Source: CAD feature listing. Evaluate the final solid. Frame: model axes, mm. Face numbers are marked on the shaded views. Coordinates: 2 decimals unless noted, no trailing zeros. Write each loop counter-clockwise with the first axis right and the second up, starting at its lowest first coordinate (ties: lowest second). Pieces come first, ordered by that corner, then holes. Notation, with made-up numbers: (-4.5, -5) -> (13.5, -5) arc R18 ccw to (13.5, 6) -> close; hole circle Ø5 at (63.5, 20). An arc over 180 degrees is marked (long way). One line per item, written item: value. Start each with the question number.
1. Line query: line 1 (Y direction, x = 10, z = -1.8); line 2 (Y direction, x = 8.5, z = -4.65); line 3 (X direction, y = 63.5, z = -1.05). Output: solid intervals per line, ascending.
2. First-contact query: P1, Ø3.5, axis at x = 10, y = 87.5, coming from the +Z side. Flat tip, straight axial feed; report the tip coordinate or a pass-through.
3. Section query D-D, the plane y = 62.5. Output: boundary loops of the cut face in (x, z).
4. Section query B-B, the plane x = 10. Output: boundary loops of the cut face in (y, z), and give its area (3 significant figures).
5. Mould query, pull axis Y, two halves, no side actions, for the marked faces 1, 2, 3 and 4. Classes: released by +Y, released by -Y, zero draft, split by the parting line, or undercut.
6. Section query C-C, the plane z = -1.5. Output: boundary loops of the cut face in (x, y), and give its area (3 significant figures).
7. Section query A-A, the plane y = 12.5. Output: boundary loops of the cut face in (x, z).
from build123d import *

# Parameters (mm, degrees)
ESQUISSE1_W        = 20
ESQUISSE1_H        = 100
ESQUISSE1_R        = 4.5
ESQUISSE1_R_2      = 2.75
BOSS_EXTRU_2_DEPTH = 5


with BuildPart() as part:
    # Esquisse1 → Boss.-Extru.2 (new body)
    # profile 1 of 3: a face of its own
    with BuildSketch(Plane.XY):
        with Locations((10, 50)):
            Rectangle(ESQUISSE1_W, ESQUISSE1_H)
        with Locations((10, 37.5)):
            Circle(ESQUISSE1_R, mode=Mode.SUBTRACT)
        with Locations((10, 62.5)):
            Circle(ESQUISSE1_R, mode=Mode.SUBTRACT)
        Polygon((10, 82.881197846), (14, 85.190598923), (14, 89.809401077), (10, 92.118802154), (6, 89.809401077), (6, 85.190598923), align=None, mode=Mode.SUBTRACT)
        Polygon((10, 7.881197846), (14, 10.190598923), (14, 14.809401077), (10, 17.118802154), (6, 14.809401077), (6, 10.190598923), align=None, mode=Mode.SUBTRACT)
    # profile 2 of 3: a face of its own
    with BuildSketch(Plane.XY):
        Polygon((6, 85.190598923), (10, 82.881197846), (14, 85.190598923), (14, 89.809401077), (10, 92.118802154), (6, 89.809401077), align=None)
        with Locations((10, 87.5)):
            Circle(ESQUISSE1_R_2, mode=Mode.SUBTRACT)
    # profile 3 of 3: a face of its own
    with BuildSketch(Plane.XY):
        Polygon((6, 10.190598923), (10, 7.881197846), (14, 10.190598923), (14, 14.809401077), (10, 17.118802154), (6, 14.809401077), align=None)
        with Locations((10, 12.5)):
            Circle(ESQUISSE1_R_2, mode=Mode.SUBTRACT)
    extrude(amount=-BOSS_EXTRU_2_DEPTH)


solid = part.part
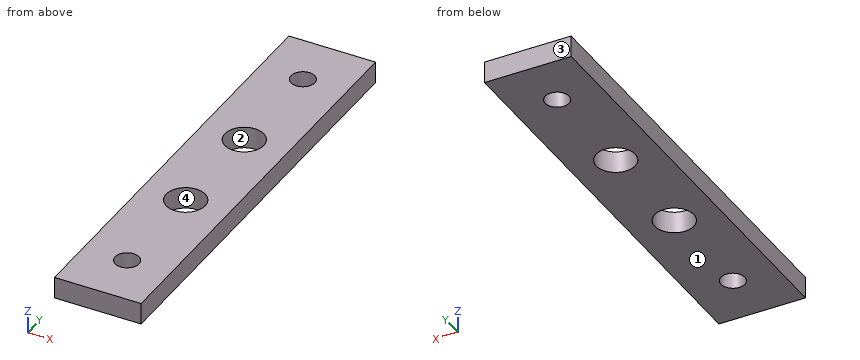
Computed values:
1. line 1: y = 0 to 9.75, 15.25 to 33, 42 to 58, 67 to 84.75, 90.25 to 100
1. line 2: y = 0 to 10.2, 14.8 to 33.26, 41.74 to 58.26, 66.74 to 85.2, 89.8 to 100
1. line 3: x = 0 to 5.61, 14.39 to 20
2. P1: passes through
3. outline: (0, -5) -> (5.5, -5) -> (5.5, 0) -> (0, 0) -> close; (14.5, -5) -> (20, -5) -> (20, 0) -> (14.5, 0) -> close
4. outline: (0, -5) -> (9.75, -5) -> (9.75, 0) -> (0, 0) -> close; (15.25, -5) -> (33, -5) -> (33, 0) -> (15.25, 0) -> close; (42, -5) -> (58, -5) -> (58, 0) -> (42, 0) -> close; (67, -5) -> (84.75, -5) -> (84.75, 0) -> (67, 0) -> close; (90.25, -5) -> (100, -5) -> (100, 0) -> (90.25, 0) -> close
4. area: 355 mm²
5. face 1: zero draft
5. face 2: undercut
5. face 3: released by +Y
5. face 4: undercut
6. outline: (0, 0) -> (20, 0) -> (20, 100) -> (0, 100) -> close; hole circle Ø9 at (10, 37.5); hole circle Ø9 at (10, 62.5); hole circle Ø5.5 at (10, 12.5); hole circle Ø5.5 at (10, 87.5)
6. area: 1,830 mm²
7. outline: (0, -5) -> (7.25, -5) -> (7.25, 0) -> (0, 0) -> close; (12.75, -5) -> (20, -5) -> (20, 0) -> (12.75, 0) -> close
